```python
from build123d import *

# Parameters (mm, degrees)
CUT_EXTRUDE1_DEPTH = 10.992209668


with BuildPart() as part:
    # Sketch1 → Revolve1 (revolve)
    with BuildSketch(Plane.XY, mode=Mode.PRIVATE) as revolve1_sk:
        with BuildLine():
            Line((0, 2), (-5, 2))
            ThreePointArc((-5, 2), (-5.707106781, 1.707106781), (-6, 1))
            Line((-6, 1), (-6, 0))
            Line((-6, 0), (0, 0))
            Line((0, 0), (0, 2))
        make_face()
    revolve(revolve1_sk.sketch.rotate(Axis((0, 2, 0), (0, -1, 0)), 270), axis=Axis((0, 2, 0), (0, -1, 0)))

    # Sketch2 → Revolve2 (revolve)
    with BuildSketch(Plane.XY, mode=Mode.PRIVATE) as revolve2_sk:
        Polygon((-4.476082848, -3.5), (-3.858938415, 0), (-2.358938415, 0), (-2.976082848, -3.5), (-2.5, -5.276765377), (-4, -5.276765377), align=None)
    revolve(revolve2_sk.sketch.rotate(Axis((0, -3.5, 0), (0, 1, 0)), 270), axis=Axis((0, -3.5, 0), (0, 1, 0)))

    # Sketch3 → Cut-Extrude1 (cut, through all)
    with BuildSketch(Plane(origin=(0, 0, 0), x_dir=(1, 0, 0), z_dir=(0, 1, 0))):
        with BuildLine():
            Line((-4.268916085, 1.345984071), (-1.345984071, 1.345984071))
            Line((-1.345984071, 1.345984071), (-1.345984071, 4.268916085))
            ThreePointArc((-1.345984071, 4.268916085), (-3.165068535, 3.165068535), (-4.268916085, 1.345984071))
        make_face()
        with BuildLine():
            Line((1.345984071, 1.345984071), (4.268916085, 1.345984071))
            ThreePointArc((4.268916085, 1.345984071), (3.165068535, 3.165068535), (1.345984071, 4.268916085))
            Line((1.345984071, 4.268916085), (1.345984071, 1.345984071))
        make_face()
        with BuildLine():
            Line((-1.345984071, -1.345984071), (-4.268916085, -1.345984071))
            ThreePointArc((-4.268916085, -1.345984071), (-3.165068535, -3.165068535), (-1.345984071, -4.268916085))
            Line((-1.345984071, -4.268916085), (-1.345984071, -1.345984071))
        make_face()
        with BuildLine():
            Line((1.345984071, -1.345984071), (1.345984071, -4.268916085))
            ThreePointArc((1.345984071, -4.268916085), (3.165068535, -3.165068535), (4.268916085, -1.345984071))
            Line((4.268916085, -1.345984071), (1.345984071, -1.345984071))
        make_face()
    extrude(amount=-CUT_EXTRUDE1_DEPTH, mode=Mode.SUBTRACT)


solid = part.part
```
The listing builds one solid part. Answer for the finished solid, in the listing's coordinates (mm). A direction names the side the tool comes from. Coordinates: 2 decimals unless noted, no trailing zeros. Loops run counter-clockwise (first coordinate to the right, second up) from the corner with the lowest first, then second, coordinate; pieces in that order, holes last. Notation, with made-up numbers: M 81.5,-21 L 111.5,-21 A27 ccw 111.5,15 Z; hole C -34,-30 d4. An arc over 180 degrees is marked long. Answer as CSV lines item,"result". Start each with the question number.
(1) Find the intervals of material crossed by L1, parallel to Y at x = 5.25, z = 1; L2, parallel to Y at x = 1.75, z = 0.5; L3, parallel to X at y = -1.25, z = -3, in increasing order. Write a range as [from, to].
(2) The mould has two halves that part along X. Classify faces 1 (the conical face through (-2.735, -4.401, -0.022)), 2 (the flat face through (-1.346, -3, -3)), 3 (the conical face through (-0.02, -4.38, 4.24)): pulls with the +X half, pulls with the -X half, needs draft (parallel to the pull), parting line crosses it, or undercut.
(3) The part is cut by section A-A (y = -2.75). Give the vertices of the cut face in (x, z).
(4) The part is cut by section C-C (z = 0). Give the vertices of the cut face in (x, y).
(5) Given pin 1 (0.7 mm diameter, centred on x = 2.5, y = -4, fed in from -Z); pin 2 (1.9 mm diameter, centred on y = -1.5, z = -2.5, fed in from -X); pin 3 (1.2 mm diameter, centred on x = -3, y = -1.5, fed in from +Z), each flat-ended and moving along its own axis, determine where each tip first touches the part or whether it passes through.
(6) For faces 4 (the conical face through (-0.021, -1.725, 4.163)), 5 (the conical face through (-4.163, -1.725, -0.021)), 6 (the conical face through (-0.02, -1.77, 2.67)), determine the directions among +Z, -Z, +X, -X, +Y, -Y from which every point of the face is accessible in a straight line to the end or side of a thin tool.
(7) The part is cut by section B-B (x = 0). Give the vertices of the cut face in (y, z).
(8) The part is cut by section D-D (y = 0.25). Give the vertices of the cut face in (x, z).
Determined:
1,L1,"[0, 1.94]"
1,L2,"[0, 2]"
1,L3,"[-1.35, 1.35]"
2,face 1,"undercut"
2,face 2,"pulls with the -X half"
2,face 3,"parting line crosses it"
3,outline,"M -4.13,-1.35 L -2.51,-1.35 A2.84 cw -2.51,1.35 L -4.13,1.35 A4.34 ccw Z; M -1.35,-4.13 A4.34 ccw 1.35,-4.13 L 1.35,-2.51 A2.84 cw -1.35,-2.51 Z; M -1.35,2.51 A2.84 cw 1.35,2.51 L 1.35,4.13 A4.34 ccw -1.35,4.13 Z; M 2.51,-1.35 L 4.13,-1.35 A4.34 ccw 4.13,1.35 L 2.51,1.35 A2.84 cw Z"
4,outline,"M -6,0 L -3.86,0 L -4.48,-3.5 L -4,-5.28 L -2.5,-5.28 L -2.98,-3.5 L -2.36,0 L 2.36,0 L 2.98,-3.5 L 2.5,-5.28 L 4,-5.28 L 4.48,-3.5 L 3.86,0 L 6,0 L 6,1 A1 ccw 5,2 L -5,2 A1 ccw -6,1 Z"
5,pin 1,"z = -1.35"
5,pin 2,"x = -1.35"
5,pin 3,"z = 1.35"
6,face 4,"+Z"
6,face 5,"-X"
6,face 6,"none"
7,outline,"M -5.28,-4 L -3.5,-4.48 L 0,-3.86 L 0,-6 L 1,-6 A1 ccw 2,-5 L 2,5 A1 ccw 1,6 L 0,6 L 0,3.86 L -3.5,4.48 L -5.28,4 L -5.28,2.5 L -3.5,2.98 L 0,2.36 L 0,-2.36 L -3.5,-2.98 L -5.28,-2.5 Z"
8,outline,"C 0,0 d12"
